Could you check a few things on this model? Use its own coordinates, in mm. Coordinates: 2 decimals unless noted, no trailing zeros. Loops run counter-clockwise (first coordinate to the right, second up) from the corner with the lowest first, then second, coordinate; pieces in that order, holes last. Notation, with made-up numbers: (24.5, -24) - (54.5, -24) arc R9 cw to (54.5, -11) - close; hole circle Ø8 at (56.5, 80.25). An arc over 180 degrees is marked (long way). One line per item, written item: value. Start each with the question number.
(1) I'm going to push flat-ended pins straight in: P1, Ø5, axis at y = 32, z = 23, coming from the -X side; P2, Ø1.5, axis at x = 3, y = 94, coming from the +Z side. Where does each tip first touch, or does it pass through?
(2) If we section it at A-A on y = 95: Write out the boundary of the cut face in (x, z).
(3) If we section it at B-B on y = 67.5: Write out the boundary of the cut face in (x, z).
(4) If I drill on line 1 along Z through (x, y) = (0, 2.15); line 2 along X through (y, z) = (101, 31.5); line 3 along X through (y, z) = (14, 35.5), over which ranges is the centre line in solid material (lowest first)? Write a range as from..to.
(5) If we mould it in two halves opening along Z, with no side actions, what happens to faces 1 (the face through (-32.17, 2.16, 36.6)), 2 (the face through (-18, 105.656, -17)), 3 (the face through (-4.33, 24.75, -21.05))? For each: pulls with the +Z half, pulls with the -Z half, needs draft (parallel to the pull), parting line crosses it, or undercut.
```python
from build123d import *

# Parameters (mm, degrees)
SKETCH1_R               = 1.016
SKETCH1_R_2             = 1.5875
SKETCH1_W               = 30.226
SKETCH1_H               = 1.016
BOSS_EXTRUDE1_DEPTH     = 1.778
CUT_EXTRUDE1_DEPTH      = 220.775953397
CUT_EXTRUDE1_DEPTH_BACK = 220.775953397
CUT_EXTRUDE2_DEPTH      = 2.54
CUT_EXTRUDE2_DEPTH_BACK = 2.54
SKETCH10_R              = 0.762
SKETCH13_R              = 43.703973106
CUT_EXTRUDE4_DEPTH      = 126


with BuildPart() as part:
    # Sketch1 → Boss-Extrude1 (new body)
    with BuildSketch(Plane(origin=(0, 0, 0), x_dir=(1, 0, 0), z_dir=(0, 1, 0))):
        with BuildLine():
            Line((19.797340731, -27.686), (33.875449694, -3.302))
            ThreePointArc((33.875449694, -3.302), (33.875449694, 19.558), (14.078108964, 30.988))
            Line((14.078108964, 30.988), (-14.078108964, 30.988))
            ThreePointArc((-14.078108964, 30.988), (-33.875449694, 19.558), (-33.875449694, -3.302))
            Line((-33.875449694, -3.302), (-19.797340731, -27.686))
            ThreePointArc((-19.797340731, -27.686), (0, -39.116), (19.797340731, -27.686))
        make_face()
        with Locations(Location((0, 10.668, 0), (0, 0, 270))):
            Circle(SKETCH1_R, mode=Mode.SUBTRACT)
        with Locations(Location((9.238759008, -5.334, 0), (0, 0, 270))):
            Circle(SKETCH1_R, mode=Mode.SUBTRACT)
        with Locations(Location((-9.238759008, -5.334, 0), (0, 0, 270))):
            Circle(SKETCH1_R, mode=Mode.SUBTRACT)
        with Locations(Location((0, 0, 0), (0, 0, 270))):
            Circle(SKETCH1_R_2, mode=Mode.SUBTRACT)
        with Locations((0, 27.94)):
            Rectangle(SKETCH1_W, SKETCH1_H, mode=Mode.SUBTRACT)
        Polygon((32.193190687, -1.135758073), (31.313308877, -0.627758073), (16.200308877, -26.804241927), (17.080190687, -27.312241927), align=None, mode=Mode.SUBTRACT)
        Polygon((-17.080190687, -27.312241927), (-16.200308877, -26.804241927), (-31.313308877, -0.627758073), (-32.193190687, -1.135758073), align=None, mode=Mode.SUBTRACT)
    extrude(amount=BOSS_EXTRUDE1_DEPTH)

    # Sweep1: sweep along a path in Sketch3
    with BuildLine(Plane(origin=(0, 1.778, 0), x_dir=(1, 0, 0), z_dir=(0, 1, 0))) as sweep1_path:
        CenterArc((0, -11.938), 39.878, 0, 360)
    # Sketch4 → Sweep1 (sweep)
    with BuildSketch(Plane(origin=(0, 0, 0), x_dir=(0, 0, -1), z_dir=(1, 0, 0))):
        Polygon((28.598946584, 0), (28.598946584, 2.534258856), (22.248946584, 7.034258856), (28.598946584, 11.534258856), (22.248946584, 16.034258856), (28.598946584, 20.534258856), (22.248946584, 25.034258856), (28.598946584, 29.534258856), (22.248946584, 34.034258856), (28.598946584, 38.534258856), (22.248946584, 43.034258856), (28.598946584, 47.534258856), (22.248946584, 52.034258856), (28.598946584, 56.534258856), (22.248946584, 61.034258856), (28.598946584, 65.534258856), (22.248946584, 70.034258856), (28.598946584, 74.534258856), (22.248946584, 79.034258856), (28.598946584, 83.534258856), (22.248946584, 88.034258856), (28.598946584, 92.534258856), (22.248946584, 97.034258856), (28.598946584, 101.534258856), (22.248946584, 106.034258856), (28.598946584, 110.534258856), (22.248946584, 115.034258856), (28.598946584, 119.534258856), (22.248946584, 124.034258856), (28.598946584, 128.534258856), (22.248946584, 133.034258856), (28.598946584, 137.534258856), (22.248946584, 142.034258856), (28.598946584, 146.534258856), (22.248946584, 151.034258856), (28.598946584, 155.534258856), (22.248946584, 160.034258856), (28.598946584, 164.534258856), (22.248946584, 169.034258856), (28.598946584, 173.534258856), (22.248946584, 178.034258856), (28.598946584, 182.534258856), (22.248946584, 187.034258856), (28.598946584, 191.534258856), (22.248946584, 196.034258856), (28.598946584, 200.534258856), (22.248946584, 205.034258856), (28.598946584, 209.534258856), (27.281053416, 209.534258856), (20.931053416, 205.034258856), (27.281053416, 200.534258856), (20.931053416, 196.034258856), (27.281053416, 191.534258856), (20.931053416, 187.034258856), (27.281053416, 182.534258856), (20.931053416, 178.034258856), (27.281053416, 173.534258856), (20.931053416, 169.034258856), (27.281053416, 164.534258856), (20.931053416, 160.034258856), (27.281053416, 155.534258856), (20.931053416, 151.034258856), (27.281053416, 146.534258856), (20.931053416, 142.034258856), (27.281053416, 137.534258856), (20.931053416, 133.034258856), (27.281053416, 128.534258856), (20.931053416, 124.034258856), (27.281053416, 119.534258856), (20.931053416, 115.034258856), (27.281053416, 110.534258856), (20.931053416, 106.034258856), (27.281053416, 101.534258856), (20.931053416, 97.034258856), (27.281053416, 92.534258856), (20.931053416, 88.034258856), (27.281053416, 83.534258856), (20.931053416, 79.034258856), (27.281053416, 74.534258856), (20.931053416, 70.034258856), (27.281053416, 65.534258856), (20.931053416, 61.034258856), (27.281053416, 56.534258856), (20.931053416, 52.034258856), (27.281053416, 47.534258856), (20.931053416, 43.034258856), (27.281053416, 38.534258856), (20.931053416, 34.034258856), (27.281053416, 29.534258856), (20.931053416, 25.034258856), (27.281053416, 20.534258856), (20.931053416, 16.034258856), (27.281053416, 11.534258856), (20.931053416, 7.034258856), (27.281053416, 2.534258856), (27.281053416, 0), align=None)
    sweep(path=sweep1_path.line)

    # Sketch5 → Cut-Extrude1 (cut, two sides: drawn at the far end of the back side and taken through both)
    with BuildSketch(Plane(origin=(0, 0, 0), x_dir=(0, 0, -1), z_dir=(1, 0, 0)).offset(-CUT_EXTRUDE1_DEPTH_BACK)):
        Polygon((-3.302, 1.778), (53.644453892, 1.778), (53.644453892, 0), (-109.531045718, -2.438778333), (-109.531045718, 1.778), (-27.686, 1.778), align=None)
    extrude(amount=CUT_EXTRUDE1_DEPTH + CUT_EXTRUDE1_DEPTH_BACK, mode=Mode.SUBTRACT)

    # Sweep2: sweep along a curve in space
    with BuildLine() as sweep2_path:
        ThreePointArc((0, 1.778, -28.598946584), (28.663949818, 1.778, -16.725949818), (40.536946584, 1.778, 11.938))
        ThreePointArc((40.536946584, 1.778, 11.938), (28.663949818, 1.778, 40.601949818), (0, 1.778, 52.474946584))
        ThreePointArc((0, 1.778, 52.474946584), (-28.663949818, 1.778, 40.601949818), (-40.536946584, 1.778, 11.938))
        ThreePointArc((-40.536946584, 1.778, 11.938), (-28.663949818, 1.778, -16.725949818), (0, 1.778, -28.598946584))
    # Sketch8 → Sweep2 (sweep)
    with BuildSketch(Plane(origin=(0, 0, 0), x_dir=(0, 0, -1), z_dir=(1, 0, 0))):
        Polygon((27.281053416, 1.778), (20.093617346, -3.453908136), (21.411510514, -3.453908136), (28.598946584, 1.778), align=None)
    sweep(path=sweep2_path.line)

    # Sketch12 → Revolve1 (revolve)
    with BuildSketch(Plane(origin=(0, 0, 0), x_dir=(0, 0, -1), z_dir=(1, 0, 0))):
        Polygon((28.598946584, 1.778), (27.281053416, 1.778), (20.093617346, -3.453908136), (21.411510514, -3.453908136), align=None)
        Polygon((20.093617346, 214.766166991), (21.411510514, 214.766166991), (28.598946584, 209.534258856), (27.281053416, 208.600318815), (27.281053416, 209.534258856), align=None)
    revolve(axis=Axis((0, 209.534258856, 11.938), (0, 1, 0)))

    # Sketch10 → Cut-Extrude2 (cut, two sides: drawn at the far end of the back side and taken through both)
    with BuildSketch(Plane(origin=(0, -12.445383757, -9.059295122), x_dir=(1, 0, 0), z_dir=(0, 0.8084854971869895, 0.5885161007468755)).offset(-CUT_EXTRUDE2_DEPTH_BACK)):
        with Locations(Location((0, 19.668215175, 0), (0, 0, 90))):
            Circle(SKETCH10_R)
    extrude(amount=CUT_EXTRUDE2_DEPTH + CUT_EXTRUDE2_DEPTH_BACK, mode=Mode.SUBTRACT)

    # Sketch13 → Cut-Extrude4 (cut)
    with BuildSketch(Plane(origin=(0, 105.656129428, 0), x_dir=(1, 0, 0), z_dir=(0, 1, 0))):
        with Locations((0, -11.938)):
            Circle(SKETCH13_R)
    extrude(amount=CUT_EXTRUDE4_DEPTH, mode=Mode.SUBTRACT)


solid = part.part
```
Values:
1. P1: stops at x = -39.11
1. P2: stops at z = 51.35
2. outline: circle Ø74.12 at (0, 11.94); hole circle Ø71.48 at (0, 11.94)
3. outline: circle Ø75.53 at (0, 11.94); hole circle Ø72.89 at (0, 11.94)
4. line 1: z = -28.6..-27.28, 51.16..52.47
4. line 2: x = -34.64..-33.12, 33.12..34.64
4. line 3: x = -28.6..-26.87, 26.87..28.6
5. face 1: parting line crosses it
5. face 2: needs draft
5. face 3: undercut
